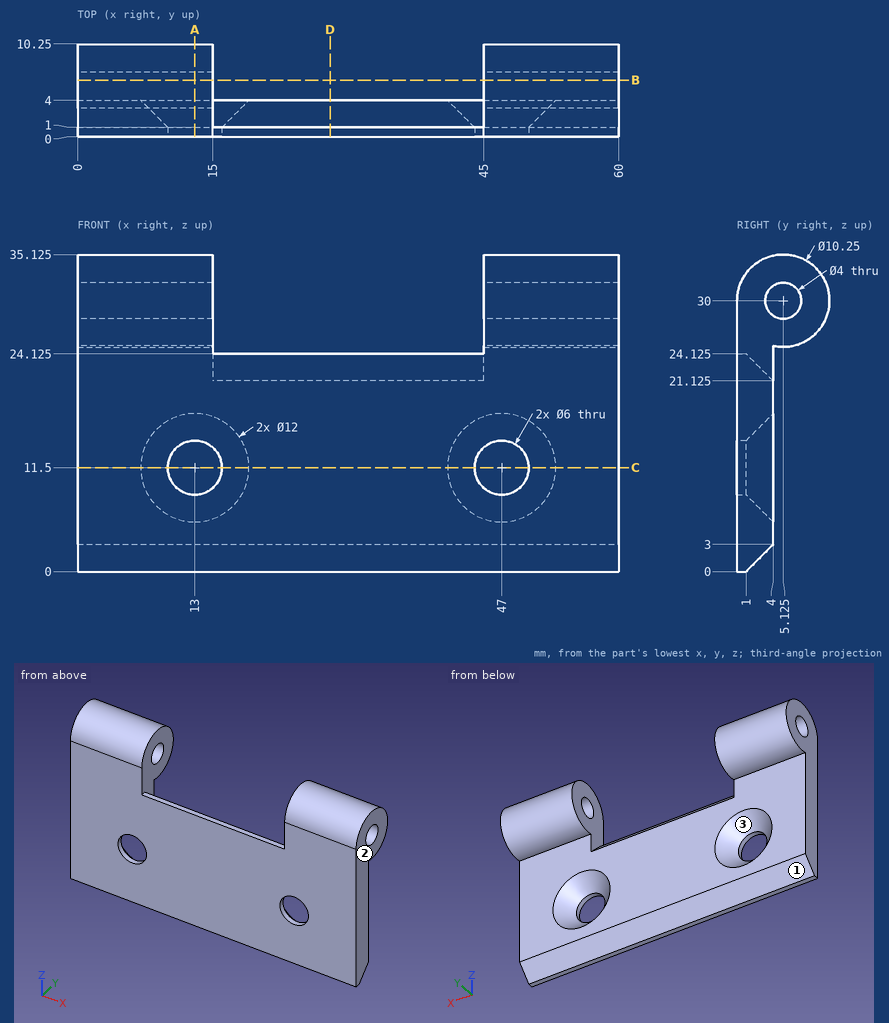
Check sheet for the drawn part. Datum: minimum x, y, z corner. Units: mm. Give positions to 0.01 mm unless a question says otherwise; leave off trailing zeros. Order: outer loops, then holes, each group sorted by start corner. A loop starts at its lowest first (then second) coordinate and runs counter-clockwise, first axis right, second up. Notation, with made-up numbers: (37.5, 65) - (70.5, 65) arc R17 ccw to (70.5, 69) - close; hole circle Ø7 at (87.5, 68.25). An arc over 180 degrees is marked (long way). Answer as a JSON object with one key per item and string values.
(1) Material ranges on line 1 (X direction, y = 0.25, z = 11.5); line 2 (Y direction, x = 52, z = 30) (3 decimals); line 3 (X direction, y = 4.75, z = 25), recorded low to high.
Report:
{"line 1": "0 to 10, 16 to 44, 50 to 60", "line 2": "0 to 3.125, 7.125 to 10.25", "line 3": "0 to 15, 45 to 60"}
(2) Cross-section at D-D (x = 28). Record the cut outline in (y, z) (3 decimals).
Report:
{"outline": "(0, 0) - (1, 0) - (4, 3) - (4, 21.125) - (1, 24.125) - (0, 24.125) - close"}
(3) Cross-section at C-C (z = 11.5). Record the cut outline in (x, y), then the cut area to 3 significant figures.
Report:
{"outline": "(0, 0) - (10, 0) - (10, 1) - (7, 4) - (0, 4) - close; (16, 0) - (44, 0) - (44, 1) - (41, 4) - (19, 4) - (16, 1) - close; (50, 0) - (60, 0) - (60, 4) - (53, 4) - (50, 1) - close", "area": "174 mm^2"}
(4) Draft check along Z on the marked faces 1, 2 and 3. Enter one of: released by +Z, released by -Z, zero draft, split by the parting line, or undercut.
Report:
{"face 1": "released by -Z", "face 2": "zero draft", "face 3": "undercut"}
(5) Cross-section at A-A (x = 13). Record the cut outline in (y, z) (3 decimals).
Report:
{"outline": "(0, 0) - (1, 0) - (4, 3) - (4, 5.5) - (1, 8.5) - (0, 8.5) - close; (0, 14.5) - (1, 14.5) - (4, 17.5) - (4, 25) arc R5.125 ccw (long way) to (0, 30) - close; hole circle Ø4 at (5.125, 30)"}
(6) Cross-section at B-B (y = 6.25). Record the cut outline in (x, z), then the cut area to 3 significant figures.
Report:
{"outline": "(0, 25) - (15, 25) - (15, 28.35) - (0, 28.35) - close; (0, 31.65) - (15, 31.65) - (15, 35) - (0, 35) - close; (45, 25) - (60, 25) - (60, 28.35) - (45, 28.35) - close; (45, 31.65) - (60, 31.65) - (60, 35) - (45, 35) - close", "area": "201 mm^2"}
(7) Depth check by flat-ended pin: pin 1 Ø17.5 at (x, z) = (38.5, 10.5) entering from +Y; pin 2 Ø0.8 at (x, y) = (24, 0.5) entering from +Z (3 decimals); pin 3 Ø2.5 at (y, z) = (5.125, 30) entering from -X. Enter the tip coordinate at first touch or a pass-through.
Report:
{"pin 1": "y = 4", "pin 2": "z = 24.125", "pin 3": "through"}
